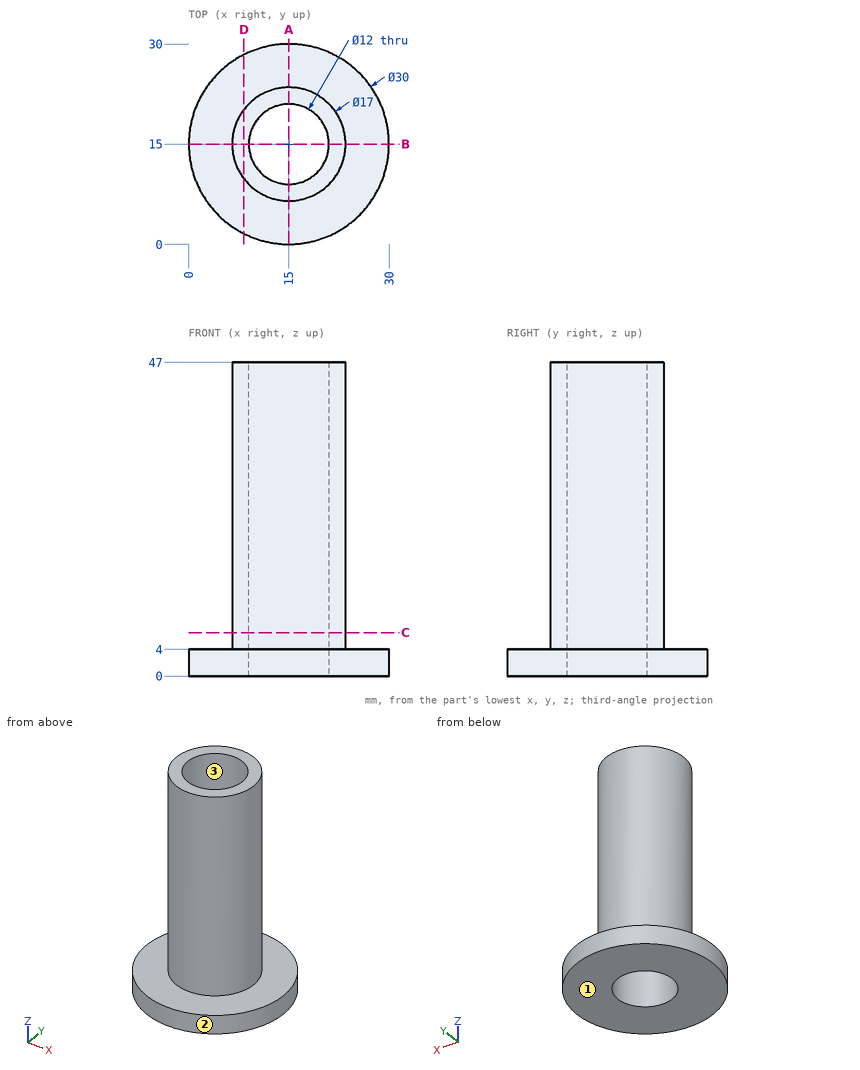
Check sheet for the drawn part. Datum: minimum x, y, z corner. Units: mm. Round coordinates to 2 decimals unless told otherwise and drop trailing zeros. Order: outer loops, then holes, each group sorted by start corner. A loop starts at its lowest first (then second) coordinate and runs counter-clockwise, first axis right, second up.
1) Section check A-A (x = 15). Record the boundary of the cut face in (y, z).
2) Scan lines: line 1 (Y direction, x = 15, z = 20); line 2 (X direction, y = 9.5, z = 44); line 3 (Z direction, x = 21.75, y = 24.25). Record each from-to range of solid material in increasing order.
3) Section check C-C (z = 6.5). Record the boundary of the cut face in (x, y).
4) Mould release check, pull along Y, two halves, no side actions. Record for the marked faces 1, 2 and 3: +Y half, -Y half, draft (parallel to the pull), parting line (faces both ways), or undercut.
5) Section check D-D (x = 8.25). Record the boundary of the cut face in (y, z), and give its area (3 significant figures).
6) Go/stop test with flat-tipped pins: pin 1 Ø15.5 at (x, y) = (15, 15) entering from -Z; pin 2 Ø1.5 at (y, z) = (15, 19.5) entering from -X; pin 3 Ø4 at (x, z) = (11, 32.5) entering from +Y; pin 4 Ø2 at (y, z) = (19.5, 24) entering from -X. Record where each tip stops, or that it passes through.
Result:
1. outline: (0, 0) - (9, 0) - (9, 47) - (6.5, 47) - (6.5, 4) - (0, 4) - close; (21, 0) - (30, 0) - (30, 4) - (23.5, 4) - (23.5, 47) - (21, 47) - close
2. line 1: y = 6.5 to 9, 21 to 23.5
2. line 2: x = 8.52 to 12.6, 17.4 to 21.48
2. line 3: z = 0 to 4
3. outline: circle Ø17 at (15, 15); hole circle Ø12 at (15, 15)
4. face 1: draft
4. face 2: parting line
4. face 3: undercut
5. outline: (1.6, 0) - (28.4, 0) - (28.4, 4) - (20.17, 4) - (20.17, 47) - (9.83, 47) - (9.83, 4) - (1.6, 4) - close
5. area: 551 mm2
6. pin 1: stops at z = 0
6. pin 2: stops at x = 6.5
6. pin 3: stops at y = 23.26
6. pin 4: stops at x = 7.25
